Build history of the part. All positions in model axes, mm. A direction names the side the tool comes from. Round coordinates to 2 decimals unless told otherwise and drop trailing zeros. Write each loop counter-clockwise with the first axis right and the second up, starting at its lowest first coordinate (ties: lowest second). Pieces come first, ordered by that corner, then holes.
Solid Edge part; units mm, degrees
sketch "Sketch1" plane through (0, 0, 0) normal (1, 0, 0) x (0, 1, 0)
  line L0 (0, 0) -> (3.9, 0)
  line L1 (3.9, 0) -> (3.9, 14)
  line L2 (3.9, 14) -> (3, 14)
  line L3 (3, 14) -> (3, 16)
  line L4 (3, 16) -> (3.9, 16)
  line L5 (3.9, 16) -> (3.9, 51.6552)
  line L6 (3.9, 51.6552) -> (3.9, 65)
  line L7 (3.9, 65) -> (6, 65)
  line L8 (6, 66) -> (6, 65)
  line L9 (4.5, 66) -> (6, 66)
  line L10 (4.5, 67) -> (4.5, 66)
  line L11 (2.5, 67) -> (4.5, 67)
  line L12 (2.5, 68) -> (2.5, 67)
  line L13 (0, 68) -> (2.5, 68)
revolve "RevolvedProtrusion1" add sketch "Sketch1" angle 360 about axis through (0, 0, 0) along (0, 0, 1)
fillet "Lekerekítés_1" radius 0.1 2 edges at (-6, 0, 66) (-6, 0, 65)
fillet "Lekerekítés_2" radius 0.1 2 edges at (-4.5, 0, 67) (-2.5, 0, 68)
properties material "Rozsdamentes acél"
1) Wall check: L1, parallel to Z at x = 0, y = 4.75; L2, parallel to Z at x = 3.25, y = -3; L3, parallel to X at y = -3, z = 5. Give the ranges that are in metal, low to high.
Results:
L1: z = 65 to 66
L2: z = 65 to 67
L3: x = -2.49 to 2.49
2) Which spindle directions (+Z, -Z, +X, -X, +Y, -Y) get a long thin tool onto all of the face, cutting with end or side? Do faces 5 (the flat face through (1, 4, 65)), 6 (the cylindrical face through (4.46, -0.59, 66.44)), 7 (the flat face through (3, 1, 16)). Say none if no direction does.
Results:
face 5: -Z
face 6: +Z
face 7: none
3) Mould opens along Z. For faces 1 (the flat face through (2, 2, 67)), 2 (the flat face through (0, 0, 0)), 3 (the flat face through (3, 1, 14)), 4 (the cylindrical face through (-2.64, -2.87, 40.84)) say: released by +Z, released by -Z, zero draft, split by the parting line, or undercut.
Results:
face 1: released by +Z
face 2: released by -Z
face 3: undercut
face 4: zero draft
4) Pin check, flat tips, straight feed: pin 1 Ø1.5 at (x, z) = (-5, 49.5) entering from +Y; pin 2 Ø1.5 at (x, z) = (-2, 36.5) entering from -Y; pin 3 Ø6 at (x, y) = (0, -1.5) entering from -Z; pin 4 Ø2 at (y, z) = (3, 48) entering from -X. Stop position of each tip, or through.
Results:
pin 1: passes through
pin 2: stops at y = -3.69
pin 3: stops at z = 0
pin 4: stops at x = -3.35
5) Slice it at C-C (z = 6.5). Write the cut outline in (x, y).
Results:
outline: circle Ø7.8 at (0, 0)
